from build123d import *

# Parameters (mm, degrees)
SKETCH1_W           = 245
SKETCH1_H           = 118
BOSS_EXTRUDE1_DEPTH = 1.5
SKETCH2_W           = 37
SKETCH2_H           = 22
SKETCH2_W_2         = 66
SKETCH2_H_2         = 26
SKETCH2_W_3         = 25
SKETCH2_H_3         = 80
CUT_EXTRUDE1_DEPTH  = 2.5
SKETCH3_R           = 1.65
CUT_EXTRUDE2_DEPTH  = 10
FILLET1_R           = 4


with BuildPart() as part:
    # Sketch1 → Boss-Extrude1 (new body)
    with BuildSketch(Plane(origin=(0, 0, 0), x_dir=(1, 0, 0), z_dir=(0, 1, 0))):
        with Locations((122.5, 59)):
            Rectangle(SKETCH1_W, SKETCH1_H)
    extrude(amount=BOSS_EXTRUDE1_DEPTH)

    # Sketch2 → Cut-Extrude1 (cut, through all)
    with BuildSketch(Plane(origin=(0, 1.5, 0), x_dir=(1, 0, 0), z_dir=(0, 1, 0))):
        with Locations((18.5, 107)):
            Rectangle(SKETCH2_W, SKETCH2_H)
        with Locations((33, 13)):
            Rectangle(SKETCH2_W_2, SKETCH2_H_2)
        with Locations((226.5, 107)):
            Rectangle(SKETCH2_W, SKETCH2_H)
        with Locations((212, 13)):
            Rectangle(SKETCH2_W_2, SKETCH2_H_2)
        with Locations((122.5, 40)):
            Rectangle(SKETCH2_W_3, SKETCH2_H_3)
    extrude(amount=-CUT_EXTRUDE1_DEPTH, mode=Mode.SUBTRACT)

    # Sketch3 → Cut-Extrude2 (cut)
    with BuildSketch(Plane.XZ):
        with Locations((5, -31)):
            Circle(SKETCH3_R)
        with Locations((5, -91)):
            Circle(SKETCH3_R)
        with Locations((105, -5)):
            Circle(SKETCH3_R)
        with Locations((105, -51)):
            Circle(SKETCH3_R)
        with Locations((105, -113)):
            Circle(SKETCH3_R)
        with Locations((140, -51)):
            Circle(SKETCH3_R)
        with Locations((140, -5)):
            Circle(SKETCH3_R)
        with Locations((140, -113)):
            Circle(SKETCH3_R)
        with Locations((240, -31)):
            Circle(SKETCH3_R)
        with Locations((240, -91)):
            Circle(SKETCH3_R)
        with Locations((62, -31)):
            Circle(SKETCH3_R)
        with Locations((82, -31)):
            Circle(SKETCH3_R)
        with Locations((163, -31)):
            Circle(SKETCH3_R)
        with Locations((183, -31)):
            Circle(SKETCH3_R)
    extrude(amount=-CUT_EXTRUDE2_DEPTH, mode=Mode.SUBTRACT)

    # Fillet1
    fillet1_edges = [part.edges().sort_by_distance(p)[0] for p in [
        (0, 0.75, -26),
        (245, 0.75, -96),
        (245, 0.75, -26),
        (110, 0.75, 0),
        (135, 0.75, 0),
        (0, 0.75, -96),
    ]]
    fillet(fillet1_edges, radius=FILLET1_R)


solid = part.part
Here's how the part is built. I have some questions about the finished solid (model axes, mm). Round coordinates to 2 decimals unless told otherwise and drop trailing zeros. Order: outer loops, then holes, each group sorted by start corner. A loop starts at its lowest first (then second) coordinate and runs counter-clockwise, first axis right, second up. Notation, with made-up numbers: (25.25, 87) -> (70.25, 87) arc R23 ccw to (70.25, 101) -> close; hole circle Ø7 at (34, -16). An arc over 180 degrees is marked (long way). Return JSON: item names as keys, results as strings.
Q1. If we section it at B-B on y = 0.85: Give the number of separate pieces and of enclosed holes in the cut face, plus the area to 3 significant figures.
Filled sheet:
{"separate pieces": "1", "enclosed holes": "14", "area": "21,700 mm^2"}
Q2. I need wall thicknesses on line 1 along X through (y, z) = (1, -91); line 2 along Z through (x, y) = (240, 1); line 3 along X through (y, z) = (0.2, -36.5). Which ranges of each line are inside material? Lowest first, please. Write a range as from..to.
Filled sheet:
{"line 1": "x = 0..3.35, 6.65..238.35, 241.65..245", "line 2": "z = -96..-92.65, -89.35..-32.65, -29.35..-26", "line 3": "x = 0..110, 135..245"}
Q3. If we section it at A-A on z = -75: List the corners of the cut face in (x, y) for me.
Filled sheet:
{"outline": "(0, 0) -> (110, 0) -> (110, 1.5) -> (0, 1.5) -> close; (135, 0) -> (245, 0) -> (245, 1.5) -> (135, 1.5) -> close"}
Q4. For pin 1 Ø4 at (x, z) = (240, -91) entering from +Y; pin 2 Ø0.8 at (y, z) = (0.5, -13) entering from -X, each with a flat end and sliding along its axis, tell me the tip position at first contact or that it passes through.
Filled sheet:
{"pin 1": "stops at y = 1.5", "pin 2": "stops at x = 66"}
Q5. If we section it at C-C on x = 223.5: List the corners of the cut face in (y, z) for me.
Filled sheet:
{"outline": "(0, -96) -> (1.5, -96) -> (1.5, -26) -> (0, -26) -> close"}
